```python
from build123d import *

# Parameters (mm, degrees)
BOSS_EXTRU_1_DEPTH      = 5
ESQUISSE2_W             = 10
ESQUISSE2_H             = 5
ENL_V_MAT_EXTRU_2_DEPTH = 685.780986886


with BuildPart() as part:
    # Esquisse1 → Boss.-Extru.1 (new body)
    with BuildSketch(Plane.XY):
        Polygon((400, 20), (400, 330), (600, 330), (600, 0), (400, 0), (0, 0), (0, 20), align=None)
    extrude(amount=BOSS_EXTRU_1_DEPTH)

    # Esquisse2 → Enlèv. mat.-Extru.2 (cut, through all)
    with BuildSketch(Plane.XY.offset(5)):
        with Locations((25, 2.5)):
            Rectangle(ESQUISSE2_W, ESQUISSE2_H)
        with Locations((5, 2.5)):
            Rectangle(ESQUISSE2_W, ESQUISSE2_H)
        with Locations((45, 2.5)):
            Rectangle(ESQUISSE2_W, ESQUISSE2_H)
        with Locations((65, 2.5)):
            Rectangle(ESQUISSE2_W, ESQUISSE2_H)
        with Locations((85, 2.5)):
            Rectangle(ESQUISSE2_W, ESQUISSE2_H)
        with Locations((105, 2.5)):
            Rectangle(ESQUISSE2_W, ESQUISSE2_H)
        with Locations((125, 2.5)):
            Rectangle(ESQUISSE2_W, ESQUISSE2_H)
        with Locations((145, 2.5)):
            Rectangle(ESQUISSE2_W, ESQUISSE2_H)
        with Locations((165, 2.5)):
            Rectangle(ESQUISSE2_W, ESQUISSE2_H)
        with Locations((185, 2.5)):
            Rectangle(ESQUISSE2_W, ESQUISSE2_H)
        with Locations((205, 2.5)):
            Rectangle(ESQUISSE2_W, ESQUISSE2_H)
        with Locations((225, 2.5)):
            Rectangle(ESQUISSE2_W, ESQUISSE2_H)
        with Locations((245, 2.5)):
            Rectangle(ESQUISSE2_W, ESQUISSE2_H)
        with Locations((265, 2.5)):
            Rectangle(ESQUISSE2_W, ESQUISSE2_H)
        with Locations((285, 2.5)):
            Rectangle(ESQUISSE2_W, ESQUISSE2_H)
        with Locations((305, 2.5)):
            Rectangle(ESQUISSE2_W, ESQUISSE2_H)
        with Locations((325, 2.5)):
            Rectangle(ESQUISSE2_W, ESQUISSE2_H)
        with Locations((345, 2.5)):
            Rectangle(ESQUISSE2_W, ESQUISSE2_H)
        with Locations((365, 2.5)):
            Rectangle(ESQUISSE2_W, ESQUISSE2_H)
        with Locations((385, 2.5)):
            Rectangle(ESQUISSE2_W, ESQUISSE2_H)
        with Locations((405, 2.5)):
            Rectangle(ESQUISSE2_W, ESQUISSE2_H)
        with Locations((425, 2.5)):
            Rectangle(ESQUISSE2_W, ESQUISSE2_H)
        with Locations((445, 2.5)):
            Rectangle(ESQUISSE2_W, ESQUISSE2_H)
        with Locations((465, 2.5)):
            Rectangle(ESQUISSE2_W, ESQUISSE2_H)
        with Locations((485, 2.5)):
            Rectangle(ESQUISSE2_W, ESQUISSE2_H)
        with Locations((505, 2.5)):
            Rectangle(ESQUISSE2_W, ESQUISSE2_H)
        with Locations((525, 2.5)):
            Rectangle(ESQUISSE2_W, ESQUISSE2_H)
        with Locations((545, 2.5)):
            Rectangle(ESQUISSE2_W, ESQUISSE2_H)
        with Locations((565, 2.5)):
            Rectangle(ESQUISSE2_W, ESQUISSE2_H)
        Polygon((580, 0), (580, 5), (590, 5), (600, 5), (600, 0), (590, 0), align=None)
    extrude(amount=-ENL_V_MAT_EXTRU_2_DEPTH, mode=Mode.SUBTRACT)


solid = part.part
```
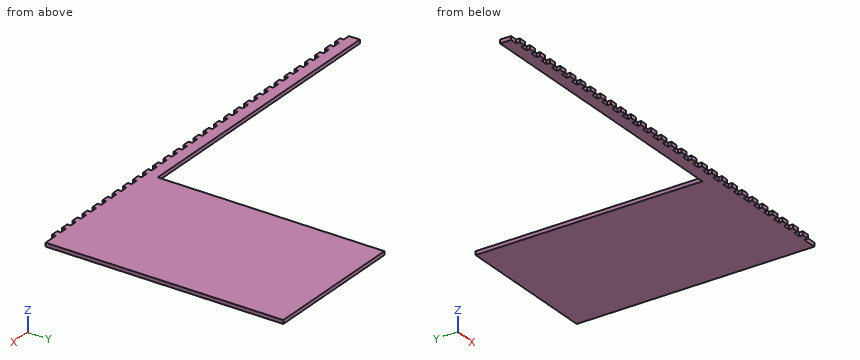
The model under review builds one solid part; all positions refer to its coordinate system, in mm. Round coordinates to 2 decimals unless told otherwise and drop trailing zeros. Loops run counter-clockwise (first coordinate to the right, second up) from the corner with the lowest first, then second, coordinate; pieces in that order, holes last.
Item 1: Clearance check with flat-ended pins moving along their axes: pin 1 Ø2 at (x, z) = (184.5, 1) entering from +Y; pin 2 Ø1.5 at (y, z) = (2.5, 2) entering from -X; pin 3 Ø1 at (y, z) = (143.5, 2) entering from -X. State where each tip first meets the part, or that it passes through.
Determined:
pin 1: stops at y = 20
pin 2: stops at x = 10
pin 3: stops at x = 400
Item 2: Take a section at A-A (y = 125). Write out the cut boundary in (x, z), then the cut area to 3 significant figures.
Determined:
outline: (400, 0) - (600, 0) - (600, 5) - (400, 5) - close
area: 1,000 mm2
Item 3: For line 1 (X direction, y = 257, z = 4.35); line 2 (Y direction, x = 267.5, z = 0.65); line 3 (Y direction, x = 391.5, z = 0.45), list the stretches that pass through material, from the lowest coordinate up.
Determined:
line 1: x = 400 to 600
line 2: y = 5 to 20
line 3: y = 0 to 20
